Geometry check sheet. Reference: the model listing, model coordinates, mm. Face numbers are marked on the shaded views. A direction names the side the tool comes from. Give positions to 0.01 mm unless a question says otherwise; leave off trailing zeros. Write each loop counter-clockwise with the first axis right and the second up, starting at its lowest first coordinate (ties: lowest second). Pieces come first, ordered by that corner, then holes. Notation, with made-up numbers: (35, 56) -> (75, 56) arc R7 cw to (75, 68) -> close; hole circle Ø10 at (56.5, 21). An arc over 180 degrees is marked (long way). Use a Markdown table: item, result. Add a question column.
Autodesk Inventor part; units mm, degrees
ref_plane "YZ Plane" through (0, 0, 0) normal (1, 0, 0) x (0, 1, 0)
ref_plane "XZ Plane" through (0, 0, 0) normal (0, 1, 0) x (-1, 0, 0)
ref_plane "XY Plane" through (0, 0, 0) normal (0, 0, 1) x (1, 0, 0)
sketch "Sketch1" plane through (0, 0, 0) normal (0, 1, 0) x (-1, 0, 0)
  line L0 (-16, 16) -> (16, 16)
  line L1 (16, 16) -> (16, -16)
  line L2 (16, -16) -> (-16, -16)
  line L3 (-16, -16) -> (-16, 16)
  line L4 (-16, 16) -> (16, -16) construction
  line L5 (16, 16) -> (-16, -16) construction
  circle A0 centre (0, 0) radius 4
  dimension "d0" = 32
  dimension "d1" = 32
  dimension "d2" = 8
extrude "Extrusion1" add sketch "Sketch1" along normal blind 4
sketch "Sketch2" plane through (0, 4, 0) normal (0, 1, 0) x (1, 0, 0)
  circle A0 centre (-8, 0) radius 2
  point P0 (0, 0)
  dimension "d5" = 4
  dimension "d6" = 8
extrude "Extrusion2" cut sketch "Sketch2" against normal blind 4
pattern_circular "Circular Pattern1" count 4 over 360 about axis through (0, 0, 0) along (0, 1, 0) of "Extrusion2"
sketch "Sketch3" plane through (0, 4, 0) normal (0, 1, 0) x (1, 0, 0)
  line L0 (-16, -16) -> (-16, 16)
  line L1 (-16, -16) -> (16, -16)
  line L2 (16, -16) -> (16, -12)
  line L3 (16, -12) -> (-16, -12)
  line L4 (-16, -12) -> (-16, -16)
  point P0 (0, 0)
  dimension "d12" = 32
  dimension "d13" = 4
extrude "Extrusion3" add sketch "Sketch3" along normal blind 32
sketch "Sketch4" plane through (16, 4, 12) normal (0, 0, -1) x (-1, 0, 0)
  line L0 (32, 0) -> (32, 32) construction
  line L1 (0, 0) -> (0, 32) construction
  circle A0 centre (16, 12) radius 4
  point P0 (16, -4)
  dimension "d16" = 8
  dimension "d26" = 32
  dimension "d27" = 12
extrude "Extrusion4" cut sketch "Sketch4" against normal blind 28
sketch "Sketch5" plane through (16, 4, 12) normal (0, 0, -1) x (-1, 0, 0)
  circle A0 centre (24, 12) radius 2
  circle A1 centre (16, 12) radius 4
  point P0 (16, -4)
  dimension "d19" = 4
  dimension "d20" = 8
extrude "Extrusion5" cut sketch "Sketch5" against normal blind 28 contours A0
pattern_circular "Circular Pattern2" count 8 over 360 about axis through (0, 16, 12) along (0, 0, 1) of "Extrusion5"
sketch "Sketch6" plane through (16, 0, 16) normal (1, 0, 0) x (0, 0, -1)
  line L0 (4, 4) -> (4, 36)
  line L1 (32, 0) -> (32, 4)
  line L2 (4, 36) -> (32, 4)
  line L3 (4, 4) -> (32, 4)
  point P0 (16, 0)
extrude "Extrusion6" add sketch "Sketch6" against normal blind 3
mirror "Mirror1" about plane through (0, 0, 0) normal (1, 0, 0) of "Extrusion6"
properties part number "KB33-046-001-002 - Уголок"
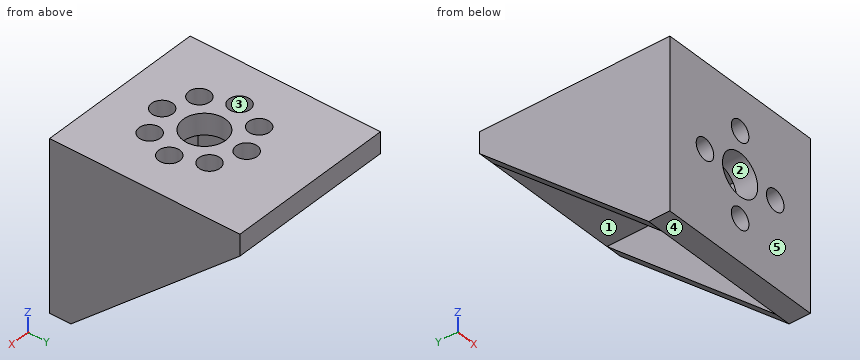
1) Gauge pin test, flat ends, axial feed: P1, Ø3.5, axis at x = 0, z = -8, coming from the +Y side; P2, Ø1, axis at x = 5.5, z = 7.5, coming from the +Y side; P3, Ø5, axis at x = 5.66, y = 21.66, coming from the -Z side. Record the tip position at first contact, or that the pin passes through.
2) Draft check along Y on the marked faces 3, 4 and 5. Enter one of: +Y half, -Y half, draft (parallel to the pull), parting line (faces both ways), or undercut.
3) Sectioned sample at B-B, the plane y = 16. Enter the section's corners in (x, z).
4) Material ranges on probe 1 along X at (y, z) = (4.5, -11); probe 2 along Z at (x, y) = (8, 1), recorded low to high. Write a range as [from, to].
5) Sectioned sample at A-A, the plane x = 0. Count the separate pieces of the cut face and the enclosed holes in it, and give its area (3 significant figures).
6) Sectioned sample at D-D, the plane x = 9.5. Enter the section's corners in (y, z).
7) Sectioned sample at C-C, the plane z = 5. Enter the section's corners in (x, y).
8) Tool access check on the marked faces 1 and 2. Record the directions out of +Z, -Z, +X, -X, +Y, -Y that give a thin tool (end or side, any length) a straight path to the whole face; none if there is none.
Check values:
| question | item | result |
|---|---|---|
| 1 | P1 | through |
| 1 | P2 | y = 4 |
| 1 | P3 | z = 12 |
| 2 | face 3 | undercut |
| 2 | face 4 | draft |
| 2 | face 5 | -Y half |
| 3 | outline | (-16, -5.5) -> (-13, -5.5) -> (-13, 12) -> (-10, 12) -> (-10, 16) -> (-16, 16) -> close; (-6, 12) -> (-4, 12) -> (-4, 16) -> (-6, 16) -> close; (4, 12) -> (6, 12) -> (6, 16) -> (4, 16) -> close; (10, 12) -> (13, 12) -> (13, -5.5) -> (16, -5.5) -> (16, 16) -> (10, 16) -> close |
| 4 | probe 1 | [-16, -13], [13, 16] |
| 4 | probe 2 | [-16, -2], [2, 16] |
| 5 | separate pieces | 7 |
| 5 | enclosed holes | 0 |
| 5 | area | 128 mm² |
| 6 | outline | (0, -16) -> (4, -16) -> (4, -1.32) -> (0, -1.32) -> close; (0, 1.32) -> (4, 1.32) -> (4, 12) -> (14.68, 12) -> (14.68, 16) -> (0, 16) -> close; (17.32, 12) -> (36, 12) -> (36, 16) -> (17.32, 16) -> close |
| 7 | outline | (-16, 0) -> (16, 0) -> (16, 28) -> (13, 28) -> (13, 4) -> (-13, 4) -> (-13, 28) -> (-16, 28) -> close |
| 8 | face 1 | -Z, +Y |
| 8 | face 2 | +Y, -Y |
